Check sheet for the modelled part. Datum: model origin and axes. Units: mm. A direction names the side the tool comes from. Round coordinates to 2 decimals unless told otherwise and drop trailing zeros. Loops run counter-clockwise (first coordinate to the right, second up) from the corner with the lowest first, then second, coordinate; pieces in that order, holes last. Notation, with made-up numbers: (72.5, -26) - (85.5, -26) arc R35 ccw to (85.5, 8) - close; hole circle Ø3 at (1, -19.75). An arc over 180 degrees is marked (long way). Put each result on its own line as item: value.
```python
from build123d import *

# Parameters (mm, degrees)
F1_DEPTH = 1.25
F2_W     = 6
F2_H     = 1
F3_DEPTH = 2.5
F4_R     = 0.75
F5_DEPTH = 75


# Not quite as in the source:
# - a feature names something its author has since deleted; it is built from what else it names


with BuildPart() as f1:
    # F0 (on Top) → F1 (new body)
    with BuildSketch(Plane.XY):
        with BuildLine():
            ThreePointArc((-7.984982332, 15.2434693582), (-9.8941706412, 14.4526576674), (-10.684982332, 12.5434693582))
            Line((-10.684982332, 12.5434693582), (-10.684982332, -6.0565306418))
            ThreePointArc((-10.684982332, -6.0565306418), (-9.8941706412, -7.965718951), (-7.984982332, -8.7565306418))
            Line((-7.984982332, -8.7565306418), (2.6008041056, -8.7565306418))
            ThreePointArc((2.6008041056, -8.7565306418), (2.983487538, -8.6804101743), (3.3079108868, -8.463637423))
            Line((3.3079108868, -8.463637423), (17.0221244492, 5.2505761394))
            ThreePointArc((17.0221244492, 5.2505761394), (17.2388972005, 5.5749994882), (17.315017668, 5.9576829206))
            Line((17.315017668, 5.9576829206), (17.315017668, 12.5434693582))
            ThreePointArc((17.315017668, 12.5434693582), (16.5242059772, 14.4526576674), (14.615017668, 15.2434693582))
            Line((14.615017668, 15.2434693582), (-7.984982332, 15.2434693582))
        make_face()
    extrude(amount=F1_DEPTH)

    # F2 (on face) → F3 (join, symmetric)
    with BuildSketch(Plane.XY.offset(1.25)):
        Polygon((-7.684982332, 12.5434693582), (-10.684982332, 12.5434693582), (-13.684982332, 12.5434693582), (-13.684982332, 11.5434693582), (-10.684982332, 11.5434693582), (-7.684982332, 11.5434693582), align=None)
        with Locations((-10.684982332, 10.0434693582)):
            Rectangle(F2_W, F2_H)
        Polygon((-13.684982332, -6.0565306418), (-10.684982332, -6.0565306418), (-7.684982332, -6.0565306418), (-7.684982332, -5.0565306418), (-10.684982332, -5.0565306418), (-13.684982332, -5.0565306418), align=None)
        with Locations((-10.684982332, -3.5565306418)):
            Rectangle(F2_W, F2_H)
    extrude(amount=F3_DEPTH, both=True)

    # F4 (on face) → F5 (cut)
    with BuildSketch(Plane.XZ.offset(6.0565306418)):
        with BuildLine():
            Line((-11.7352277888, 2.4365543881), (-7.684982332, 1.25))
            Line((-7.684982332, 1.25), (-7.684982332, 3.75))
            Line((-7.684982332, 3.75), (-13.684982332, 3.75))
            Line((-13.684982332, 3.75), (-13.684982332, -1.25))
            Line((-13.684982332, -1.25), (-7.684982332, -1.25))
            Line((-7.684982332, -1.25), (-7.684982332, 0))
            Line((-7.684982332, 0), (-10.684982332, 0))
            Line((-10.684982332, 0), (-12.0847867802, 0))
            ThreePointArc((-12.0847867802, 0), (-13.3155374428, 1.4199208375), (-11.7352277888, 2.4365543881))
        make_face()
        with Locations((-12.0847867802, 1.2433518423)):
            Circle(F4_R)
    extrude(amount=-F5_DEPTH, mode=Mode.SUBTRACT)


solid = f1.part
```
Item 1: Release check for a two-part mould opening along X. For faces 1 (the flat face through (-9.74, 10.04, 1.85)), 2 (the cylindrical face through (-12.68, 10.04, 0.79)), 3 (the flat face through (-10.685, 3, 1)) record: +X half, -X half, draft (parallel to the pull), parting line (faces both ways), or undercut.
Filled sheet:
face 1: +X half
face 2: undercut
face 3: -X half
Item 2: Section check C-C on x = -2. Enter the section's corners in (y, z), then the cut area to 3 significant figures.
Filled sheet:
outline: (-8.76, 0) - (15.24, 0) - (15.24, 1.25) - (-8.76, 1.25) - close
area: 30.0 mm²
Item 3: Section check B-B on y = 6.5. Enter the section's corners in (x, z), then the cut area to 3 significant figures.
Filled sheet:
outline: (-10.68, 0) - (17.32, 0) - (17.32, 1.25) - (-10.68, 1.25) - close
area: 35.0 mm²
Item 4: Go/stop test with flat-tipped pins: pin 1 (1.2 mm diameter, centred on x = -11, z = 1, fed in from -Y); pin 2 (4 mm diameter, centred on x = -2.5, y = -5.5, fed in from -Z); pin 3 (6 mm diameter, centred on x = 14, y = 6.5, fed in from +Z); pin 4 (1 mm diameter, centred on y = 5.5, z = 2, fed in from +X). Record where each tip stops, or that it passes through.
Filled sheet:
pin 1: y = -7.26
pin 2: z = 0
pin 3: z = 1.25
pin 4: through
Item 5: Thickness scan on line 1 (Z direction, x = -3, y = -1); line 2 (X direction, y = 6.5, z = 1); line 3 (Y direction, x = 16, z = 0.5). Record the ranges inside material, lowest first. Write a range as from..to.
Filled sheet:
line 1: 0..1.25
line 2: -10.68..17.32
line 3: 4.23..14.86
Item 6: Tool access check on faces 4 (the flat face through (-11, 10.543, 1)), 5 (the flat face through (-9.74, -3.56, 1.85)), 6 (the flat face through (-11, 12.543, 1)), 7 (the cylindrical face through (-9.92, -7.94, 0.62)), 8 (the flat face through (-10.685, 11, 1)). Record the directions out of +Z, -Z, +X, -X, +Y, -Y that give a thin tool (end or side, any length) a straight path to the whole face; none if there is none.
Filled sheet:
face 4: +Z, -X
face 5: +Z, +X, +Y, -Y
face 6: +Z, -X, +Y
face 7: +Z, -Z, -X, -Y
face 8: +Z, -Z, -X
Item 7: Section check A-A on x = -11. Enter the section's corners in (y, z).
Filled sheet:
outline: (-6.06, 0) - (-5.06, 0) - (-5.06, 2.22) - (-6.06, 2.22) - close; (-4.06, 0) - (-3.06, 0) - (-3.06, 2.22) - (-4.06, 2.22) - close; (9.54, 0) - (10.54, 0) - (10.54, 2.22) - (9.54, 2.22) - close; (11.54, 0) - (12.54, 0) - (12.54, 2.22) - (11.54, 2.22) - close
